Read the model definition and answer for the solid it produces. Units are mm, in the model's axes. A direction names the side the tool comes from. Give positions to 0.01 mm unless a question says otherwise; leave off trailing zeros. Order: outer loops, then holes, each group sorted by start corner. A loop starts at its lowest first (then second) coordinate and runs counter-clockwise, first axis right, second up. Notation, with made-up numbers: (37, 77.5) - (86, 77.5) arc R20 cw to (86, 109.5) - close; hole circle Ø11 at (28, 85.5). An arc over 180 degrees is marked (long way). Write each question's results on one line, items separated by ' | '. Start each with the question number.
Q1. Find section C-C on y = 52. Give the vertices of the cut face in (x, z).
Q2. A tool of negligible diameter and unlimited length cuts with its end or side. For faces 4 (the face through (-112, 43.738, 150)), 5 (the face through (-147.522, 58, 150)), from which of +Z, -Z, +X, -X, +Y, -Y can it reach the whole face along a straight path? Write none if from no direction.
Q3. Flat-ended cylindrical pins translate along their axes: P1, Ø1, axis at x = -103, z = 98.5, coming from the +Y side; P2, Ø6, axis at x = -98.5, y = 51.5, coming from the +Z side; P3, Ø10, axis at y = 52.5, z = 70.5, coming from the +X side. Find the tip coordinate at first contact, or state that the pin passes through.
Q4. Find section B-B on x = -130. Give the vertices of the cut face in (y, z), and give its area (3 significant figures).
Q5. Find the intervals of material crossed by line 1 along Y through (x, z) = (-127, 148); line 2 along X through (y, z) = (65.25, 107.5), in increasing order. Write a range as from..to.
Q6. For a pull along Z with two mould halves and no side action, classify faces 1 (the face through (-121, 46, 0)), 2 (the face through (-110, 46.913, 150)), 3 (the face through (-121, 46, 304.8)) as +Z half, -Z half, draft (parallel to the pull), parting line (faces both ways), or undercut.
Q7. Find section A-A on z = 254.5. Give the vertices of the cut face in (x, y).
Autodesk Inventor part; units mm, degrees
ref_plane "YZ Plane" through (0, 0, 0) normal (1, 0, 0) x (0, 1, 0)
ref_plane "XZ Plane" through (0, 0, 0) normal (0, 1, 0) x (-1, 0, 0)
ref_plane "XY Plane" through (0, 0, 0) normal (0, 0, 1) x (1, 0, 0)
sketch "Sketch1" plane through (0, 0, 0) normal (0, 0, 1) x (1, 0, 0)
  line L0 (-150.6966, 69.1379) -> (-147.5216, 69.1379)
  line L1 (-147.5216, 69.1379) -> (-147.5216, 43.7379)
  line L2 (-147.5216, 43.7379) -> (-150.6966, 43.7379)
  line L3 (-150.6966, 43.7379) -> (-150.6966, 69.1379)
  line L4 (-150.6966, 43.7379) -> (-74.4966, 43.7379)
  line L5 (-74.4966, 43.7379) -> (-74.4966, 46.9129)
  line L6 (-74.4966, 46.9129) -> (-150.6966, 46.9129)
  line L7 (-150.6966, 46.9129) -> (-150.6966, 43.7379)
  point P0 (0, 0)
  point P1 (-147.5216, 46.9129)
  dimension "d0" = 3.175
  dimension "d1" = 25.4
  dimension "d2" = 76.2
  dimension "d3" = 3.175
extrude "Extrusion1" add sketch "Sketch1" along normal blind 304.8
properties part number "shootingGuide"
Working result:
1) outline: (-150.7, 0) - (-147.52, 0) - (-147.52, 304.8) - (-150.7, 304.8) - close
2) face 4: +Z, -Z, +X, -X, -Y | face 5: +Z, -Z, +X, +Y
3) P1: y = 46.91 | P2: through | P3: x = -147.52
4) outline: (43.74, 0) - (46.91, 0) - (46.91, 304.8) - (43.74, 304.8) - close | area: 968 mm²
5) line 1: 43.74..46.91 | line 2: -150.7..-147.52
6) face 1: -Z half | face 2: draft | face 3: +Z half
7) outline: (-150.7, 43.74) - (-74.5, 43.74) - (-74.5, 46.91) - (-147.52, 46.91) - (-147.52, 69.14) - (-150.7, 69.14) - close
